Autodesk Inventor part; units mm, degrees
ref_plane "YZ Plane" through (0, 0, 0) normal (1, 0, 0) x (0, 1, 0)
ref_plane "XZ Plane" through (0, 0, 0) normal (0, 1, 0) x (-1, 0, 0)
ref_plane "XY Plane" through (0, 0, 0) normal (0, 0, 1) x (1, 0, 0)
sketch "Sketch1" plane through (0, 0, 0) normal (0, 0, 1) x (1, 0, 0)
  line L0 (0, 0) -> (14, 0)
  line L1 (14, 0) -> (14, -12)
  line L2 (14, -12) -> (0, -12)
  line L3 (0, -12) -> (0, 0)
  dimension "d0" = 14
  dimension "d1" = 12
extrude "Extrusion1" add sketch "Sketch1" against normal blind 22
sketch "Sketch2" plane through (0, 0, 0) normal (0, 0, 1) x (1, 0, 0)
  line L0 (2, -2) -> (12, -2)
  line L1 (12, -2) -> (12, -22)
  line L2 (12, -22) -> (2, -22)
  line L3 (2, -22) -> (2, -2)
  point P0 (0, 0)
  dimension "d4" = 10
  dimension "d5" = 20
extrude "Extrusion2" cut sketch "Sketch2" against normal blind 20
sketch "Sketch8" plane through (0, -12, 0) normal (-1, 0, 0) x (0, 0, 1)
  point P0 (0, 12)
sketch "Sketch9" plane through (0, -12, 0) normal (-1, 0, 0) x (0, 0, 1)
  point P0 (0, 12)
sketch "Sketch11" plane through (0, -12, 0) normal (-1, 0, 0) x (0, 0, 1)
  point P0 (0, 12)
sketch "Sketch13" plane through (0, -12, 0) normal (-1, 0, 0) x (0, 0, 1)
  line L0 (-12.5, 10) -> (-17.5, 10)
  line L1 (-17.5, 10) -> (-17.5, -0.477)
  line L2 (-17.5, -0.477) -> (-12.5, -0.477)
  line L3 (-12.5, -0.477) -> (-12.5, 10)
  point P0 (0, 12)
  dimension "d27" = 5
extrude "Extrusion9" cut sketch "Sketch13" against normal blind 10
properties part number "housing_v05"
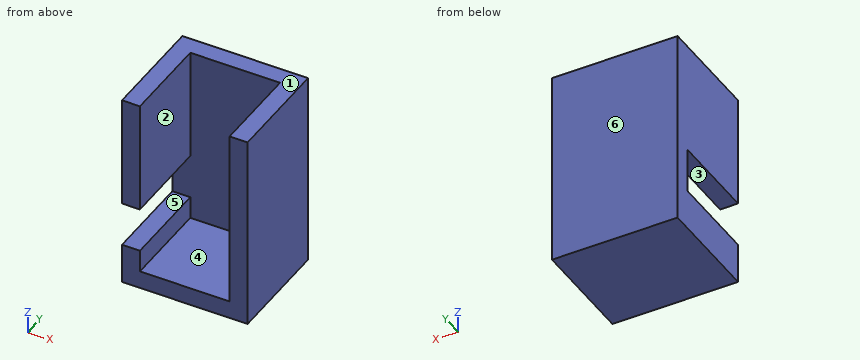
Build history of the part. All positions in model axes, mm. Face numbers are marked on the shaded views. A direction names the side the tool comes from. Round coordinates to 2 decimals unless told otherwise and drop trailing zeros. Write each loop counter-clockwise with the first axis right and the second up, starting at its lowest first coordinate (ties: lowest second). Pieces come first, ordered by that corner, then holes. Notation, with made-up numbers: (-34.5, -16.5) -> (-1.5, -16.5) arc R13 cw to (-1.5, 8.5) -> close; hole circle Ø1 at (73, 64.25). An arc over 180 degrees is marked (long way). Write item = value, one per line.
(1) Two-plate mould, pull along Z, no slides. Class the marked faces 1, 2 and 3: pulls with the +Z half, pulls with the -Z half, needs draft (parallel to the pull), parting line crosses it, or undercut.
Answer:
face_1 = pulls with the +Z half
face_2 = needs draft
face_3 = undercut
(2) Band-saw the part on A-A (y = -6). Give the cut face in (x, z), then the cut area to 3 significant figures.
Answer:
outline = (0, -22) -> (14, -22) -> (14, 0) -> (12, 0) -> (12, -20) -> (2, -20) -> (2, -17.5) -> (0, -17.5) -> close; (0, -12.5) -> (2, -12.5) -> (2, 0) -> (0, 0) -> close
area = 98.0 mm2
(3) Probe L1, parallel to X at y = -9.25, z = -3; L2, parallel to Z at x = 6, y = -3.5; L3, parallel to Y at x = 6, z = -10.25. List the from-to ranges inside material, lowest first.
Answer:
L1 = 0 to 2, 12 to 14
L2 = -22 to -20
L3 = -2 to 0
(4) Band-saw the part on B-B (x = 1.75). Give the cut face in (y, z).
Answer:
outline = (-12, -22) -> (0, -22) -> (0, 0) -> (-12, 0) -> (-12, -12.5) -> (-2, -12.5) -> (-2, -17.5) -> (-12, -17.5) -> close
(5) Tool access for the marked faces 4, 5 and 6: list every direction of +Z, -Z, +X, -X, +Y, -Y with a clear straight run to the whole face (end or side of a thin tool).
Answer:
face_4 = +Z, -Y
face_5 = -X, -Y
face_6 = +Z, -Z, +X, -X, +Y
(6) Band-saw the part on C-C (z = -11.25). Give the cut face in (x, y).
Answer:
outline = (0, -12) -> (2, -12) -> (2, -2) -> (12, -2) -> (12, -12) -> (14, -12) -> (14, 0) -> (0, 0) -> close
